The figure shows three views and two pictorial views of one solid part (mm, origin at its lowest corner). Answer the questions. A direction names the side the tool comes from. Round coordinates to 2 decimals unless told otherwise and drop trailing zeros. Write each loop counter-clockwise with the first axis right and the second up, starting at its lowest first coordinate (ties: lowest second). Pieces come first, ordered by that corner, then holes. Notation, with made-up numbers: (66.25, -21) -> (105.25, -21) arc R20 cw to (105.25, -15) -> close; hole circle Ø6 at (3.5, 6.25). An arc over 180 degrees is marked (long way). One line per item, written item: value.
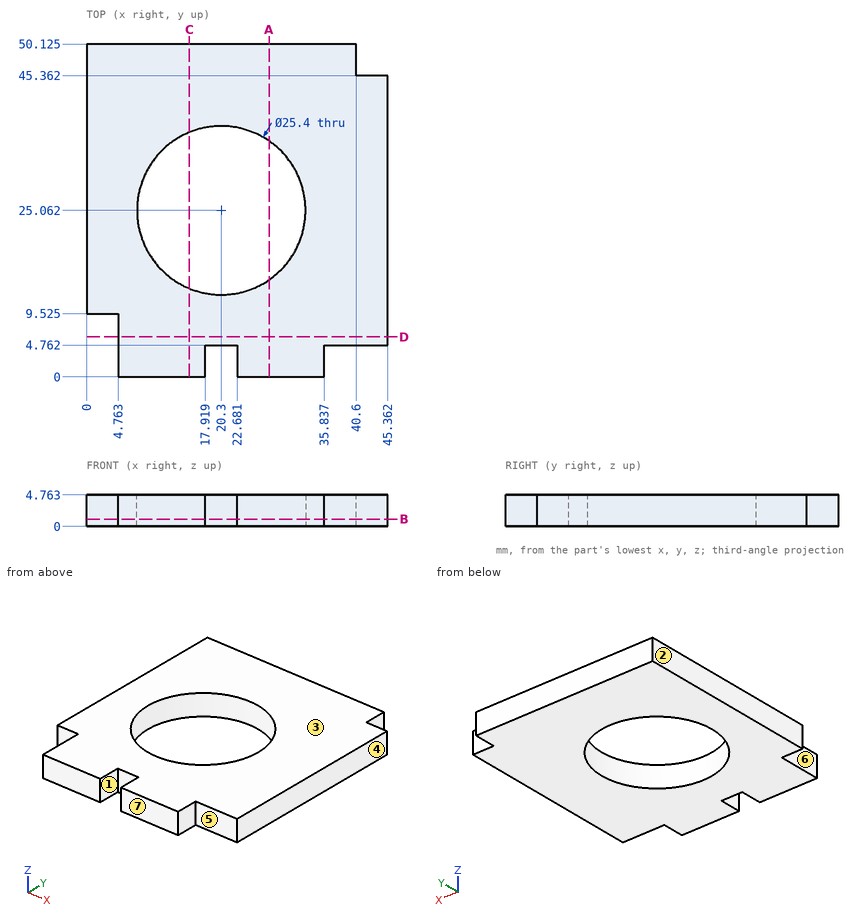
(1) For a pull along X with two mould halves and no side action, classify the marked faces 1, 2, 3 and 4 as pulls with the +X half, pulls with the -X half, needs draft (parallel to the pull), parting line crosses it, or undercut.
Reported:
face 1: undercut
face 2: pulls with the -X half
face 3: needs draft
face 4: pulls with the +X half
(2) Flat-ended cylindrical pins translate along their axes: pin 1 Ø1.4 at (y, z) = (47.5, 1.5) entering from +X; pin 2 Ø1.4 at (y, z) = (3, 1.5) entering from -X; pin 3 Ø1.4 at (y, z) = (2.5, 2) entering from +X; pin 4 Ø15 at (x, y) = (20.3, 25.06) entering from +Z. Find the tip coordinate at first contact, or state that the pin passes through.
Reported:
pin 1: stops at x = 40.6
pin 2: stops at x = 4.76
pin 3: stops at x = 35.84
pin 4: passes through
(3) A tool of negligible diameter and unlimited length cuts with its end or side. For the marked faces 5, 6 and 7, from which of +Z, -Z, +X, -X, +Y, -Y can it reach the whole face along a straight path? Write none if from no direction.
Reported:
face 5: +Z, -Z, +X, -Y
face 6: +Z, -Z, -X, -Y
face 7: +Z, -Z, +X, -X, -Y
(4) Find section C-C on x = 15.5. Give the vertices of the cut face in (y, z) (1 decimal), plus the area to 3 significant figures.
Reported:
outline: (0, 0) -> (13.3, 0) -> (13.3, 4.8) -> (0, 4.8) -> close; (36.8, 0) -> (50.1, 0) -> (50.1, 4.8) -> (36.8, 4.8) -> close
area: 127 mm2
(5) Find section B-B on z = 1.1. Give the vertices of the cut face in (x, y) (1 decimal).
Reported:
outline: (0, 9.5) -> (4.8, 9.5) -> (4.8, 0) -> (17.9, 0) -> (17.9, 4.8) -> (22.7, 4.8) -> (22.7, 0) -> (35.8, 0) -> (35.8, 4.8) -> (45.4, 4.8) -> (45.4, 45.4) -> (40.6, 45.4) -> (40.6, 50.1) -> (0, 50.1) -> close; hole circle Ø25.4 at (20.3, 25.1)
(6) Consider probe 1 along Y at (x, z) = (20.3, 2.65) (1 decimal); probe 2 along X at (y, z) = (35, 2.85) (1 decimal); probe 3 along Y at (x, z) = (3, 0.6) (1 decimal). Determine where each line is inside the solid, lowest interval first.
Reported:
probe 1: y = 4.8 to 12.4, 37.8 to 50.1
probe 2: x = 0 to 12.4, 28.2 to 45.4
probe 3: y = 9.5 to 50.1
(7) Find section A-A on x = 27.5. Give the vertices of the cut face in (y, z) (1 decimal).
Reported:
outline: (0, 0) -> (14.6, 0) -> (14.6, 4.8) -> (0, 4.8) -> close; (35.5, 0) -> (50.1, 0) -> (50.1, 4.8) -> (35.5, 4.8) -> close
(8) Find section D-D on y = 6. Give the vertices of the cut face in (x, z), plus the area to 3 significant figures.
Reported:
outline: (4.76, 0) -> (45.36, 0) -> (45.36, 4.76) -> (4.76, 4.76) -> close
area: 193 mm2
